The model under review builds one solid part; all positions refer to its coordinate system, in mm. Face numbers are marked on the shaded views. A direction names the side the tool comes from. Give positions to 0.01 mm unless a question says otherwise; leave off trailing zeros. Loops run counter-clockwise (first coordinate to the right, second up) from the corner with the lowest first, then second, coordinate; pieces in that order, holes last. Notation, with made-up numbers: M 27,-38.5 L 72,-38.5 A19 ccw 72,-12.5 Z; hole C 89.5,7 d6. An arc over 180 degrees is marked long. One line per item, written item: value. Start each with the question number.
Q1. For pin 1 (12 mm diameter, centred on x = -6, z = 40, fed in from -Y); pin 2 (8 mm diameter, centred on y = 10.5, z = 51, fed in from -X); pin 3 (5 mm diameter, centred on y = -42.5, z = 3, fed in from -X), all flat-tipped, find the tip position at first contact; note any pin that passes through.
Q2. To check wall thickness, follow line 1 along Y through (x, z) = (-37, 27); line 2 along Z through (x, y) = (-15.5, -52); line 3 along X through (y, z) = (-5, 27). State the ranges of each line that lie inside material, in increasing order. Write a range as from..to.
Q3. We need section C-C on x = -24. Write out the cut boundary in (y, z), plus the area to 3 significant figures.
Q4. For the marked faces 1, 2 and 3, list the 3-axis set-ups (+Z, -Z, +X, -X, +Y, -Y) from which the entire face can be reached by the end or side of a thin tool; tool diameter is ignored.
Q5. We need section A-A on z = 5. Write out the cut boundary in (x, y), plus the area to 3 significant figures.
Q6. We need section B-B on y = 17. Write out the cut boundary in (x, z).
Q7. We need section D-D on z = 31.5. Write out the cut boundary in (x, y).
```python
from build123d import *

# Parameters (mm, degrees)
F1_DEPTH = 45.72
F2_DEPTH = 10.16
F4_W     = 19.05
F4_H     = 25.4
F5_DEPTH = 10.16


with BuildPart() as f1:
    # F0 (on Top) → F1 (new body)
    with BuildSketch(Plane.XY):
        Polygon((-6.338918, 25.4), (-44.438918, 25.4), (-44.438918, -25.4), (-31.738918, -25.4), (-6.338918, -25.4), align=None)
    extrude(amount=F1_DEPTH)

    # F0 (on Top) → F2 (join)
    with BuildSketch(Plane.XY):
        Polygon((19.061082, -50.8), (-6.338918, -25.4), (-31.738918, -25.4), (-31.738918, -76.2), (19.061082, -76.2), align=None)
    extrude(amount=F2_DEPTH)

    # F4 (on offset) → F5 (join)
    with BuildSketch(Plane.XY.offset(45.72)):
        with Locations((-15.755231, 12.81299)):
            Rectangle(F4_W, F4_H)
    extrude(amount=F5_DEPTH)


solid = f1.part
```
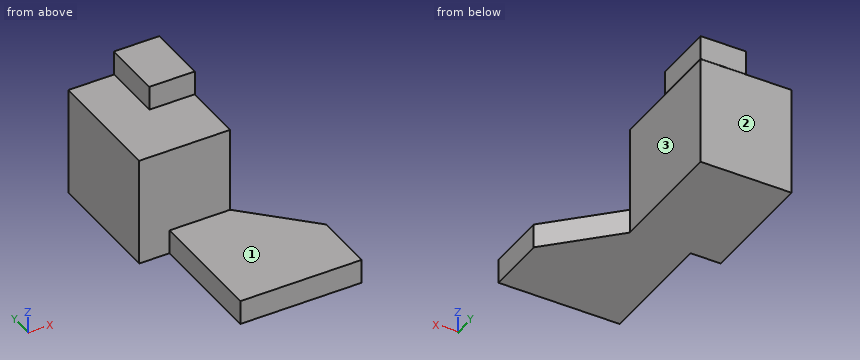
Solved:
1. pin 1: y = -25.4
1. pin 2: x = -25.28
1. pin 3: x = -31.74
2. line 1: -25.4..25.4
2. line 2: 0..10.16
2. line 3: -44.44..-6.34
3. outline: M -76.2,0 L 25.4,0 L 25.4,45.72 L 25.51,45.72 L 25.51,55.88 L 0.11,55.88 L 0.11,45.72 L -25.4,45.72 L -25.4,10.16 L -76.2,10.16 Z
3. area: 3,100 mm2
4. face 1: +Z, +X, -X, -Y
4. face 2: -Z, +X, -X, +Y
4. face 3: -Z, +X, +Y
5. outline: M -44.44,-25.4 L -31.74,-25.4 L -31.74,-76.2 L 19.06,-76.2 L 19.06,-50.8 L -6.34,-25.4 L -6.34,25.4 L -44.44,25.4 Z
5. area: 4,190 mm2
6. outline: M -44.44,0 L -6.34,0 L -6.34,45.72 L -6.23,45.72 L -6.23,55.88 L -25.28,55.88 L -25.28,45.72 L -44.44,45.72 Z
7. outline: M -44.44,-25.4 L -6.34,-25.4 L -6.34,25.4 L -44.44,25.4 Z
